Could you check a few things on this model? Use its own coordinates, in mm. A direction names the side the tool comes from. Coordinates: 2 decimals unless noted, no trailing zeros. Order: outer loops, then holes, each group sorted by start corner. A loop starts at its lowest first (then second) coordinate and runs counter-clockwise, first axis right, second up. Notation, with made-up numbers: (31.25, 51.25) -> (55.25, 51.25) arc R15 ccw to (55.25, 75.25) -> close; hole circle Ø10 at (-9, 50.25). An arc over 180 degrees is marked (long way). Return JSON: item names as keys, results as strings. Group by question number.
from build123d import *

# Parameters (mm, degrees)
CHAMFER1_SIZE         = 0.5
CHAMFER1_SIZE2        = 0.288675135
CHAMFER1_PART_2_SIZE  = 0.5
CHAMFER1_PART_2_SIZE2 = 0.288675135


with BuildPart() as part:
    # Sketch1 → Revolve1 (revolve)
    with BuildSketch(Plane.XY):
        Polygon((0, 2.38125), (0, 4.7625), (1.190625, 4.7625), (1.190625, 3.96875), (6.35, 3.96875), (6.35, 2.38125), align=None)
    revolve(axis=Axis((0, 0, 0), (1, 0, 0)))

    # Chamfer1
    chamfer1_edges = [part.edges().sort_by_distance(p)[0] for p in [
        (6.35, -2.38125, 0),
    ]]
    chamfer1_side = [part.faces().sort_by_distance(p)[0] for p in [
        (3.175, -2.38125, 0),
    ]]
    chamfer(chamfer1_edges, length=CHAMFER1_SIZE, length2=CHAMFER1_SIZE2, reference=chamfer1_side[0])

    # Chamfer1 part 2
    chamfer1_part_2_edges = [part.edges().sort_by_distance(p)[0] for p in [
        (0, -2.38125, 0),
    ]]
    chamfer1_part_2_side = [part.faces().sort_by_distance(p)[0] for p in [
        (0, -2.515953842, 0),
    ]]
    chamfer(chamfer1_part_2_edges, length=CHAMFER1_PART_2_SIZE, length2=CHAMFER1_PART_2_SIZE2, reference=chamfer1_part_2_side[0])


solid = part.part
Q1. I need wall thicknesses on line 1 along Z through (x, y) = (4.4, 0); line 2 along Y through (x, z) = (2.25, 2); line 3 along Y through (x, z) = (5.5, 1). Which ranges of each line are inside material? Lowest first, please. Write a range as from..to.
Q2. We'd pull the mould along Z, two halves only. Please class faces 3 (the cylindrical face through (3.03, -1.89, -1.45)), 4 (the flat face through (0, 0.1, -3.1)), 5 (the cylindrical face through (0.6, -3.78, -2.9)): pulls with the +Z half, pulls with the -Z half, needs draft (parallel to the pull), parting line crosses it, or undercut.
Q3. I want a section at C-C on x = 4.75. Please give me the cut outline in (y, z), and give its area (3 significant figures).
Q4. I'm going to push flat-ended pins straight in: pin 1 Ø1 at (x, z) = (0.5, -2.5) entering from -Y; pin 2 Ø2 at (x, y) = (4.5, -2) entering from +Z; pin 3 Ø1.5 at (x, y) = (4.5, 2.5) entering from +Z. Where does each tip first touch, or does it pass through?
Q5. I want a section at A-A on y = 0. Please give me the cut outline in (x, z).
Q6. On a 3-axis mill with a long thin cutter (end or side, diameter ignored), from which of +Z, -Z, +X, -X, +Y, -Y can I reach the whole of each face in a straight line? I mean faces 1 (the flat face through (6.35, 3, -1)), 2 (the cylindrical face through (3.806, -0.86, -3.874)). Say none if no direction works.
Q7. I want a section at D-D on z = -3.5. Please give me the cut outline in (x, y), and give its area (3 significant figures).
Response values:
{
 "1": {"line 1": "z = -3.97..-2.38, 2.38..3.97", "line 2": "y = -3.43..-1.29, 1.29..3.43", "line 3": "y = -3.84..-2.16, 2.16..3.84"},
 "2": {"face 3": "undercut", "face 4": "needs draft", "face 5": "parting line crosses it"},
 "3": {"outline": "circle Ø7.94 at (0, 0); hole circle Ø4.76 at (0, 0)", "area": "31.7 mm²"},
 "4": {"pin 1": "stops at y = -4.32", "pin 2": "stops at z = 3.84", "pin 3": "stops at z = 3.56"},
 "5": {"outline": "(0, -4.76) -> (1.19, -4.76) -> (1.19, -3.97) -> (6.35, -3.97) -> (6.35, -2.67) -> (5.85, -2.38) -> (0.29, -2.38) -> (0, -2.88) -> close; (0, 2.88) -> (0.29, 2.38) -> (5.85, 2.38) -> (6.35, 2.67) -> (6.35, 3.97) -> (1.19, 3.97) -> (1.19, 4.76) -> (0, 4.76) -> close"},
 "6": {"face 1": "+Z, -Z, +X, +Y, -Y", "face 2": "+X"},
 "7": {"outline": "(0, -3.23) -> (1.19, -3.23) -> (1.19, -1.87) -> (6.35, -1.87) -> (6.35, 1.87) -> (1.19, 1.87) -> (1.19, 3.23) -> (0, 3.23) -> close", "area": "27.0 mm²"}
}
